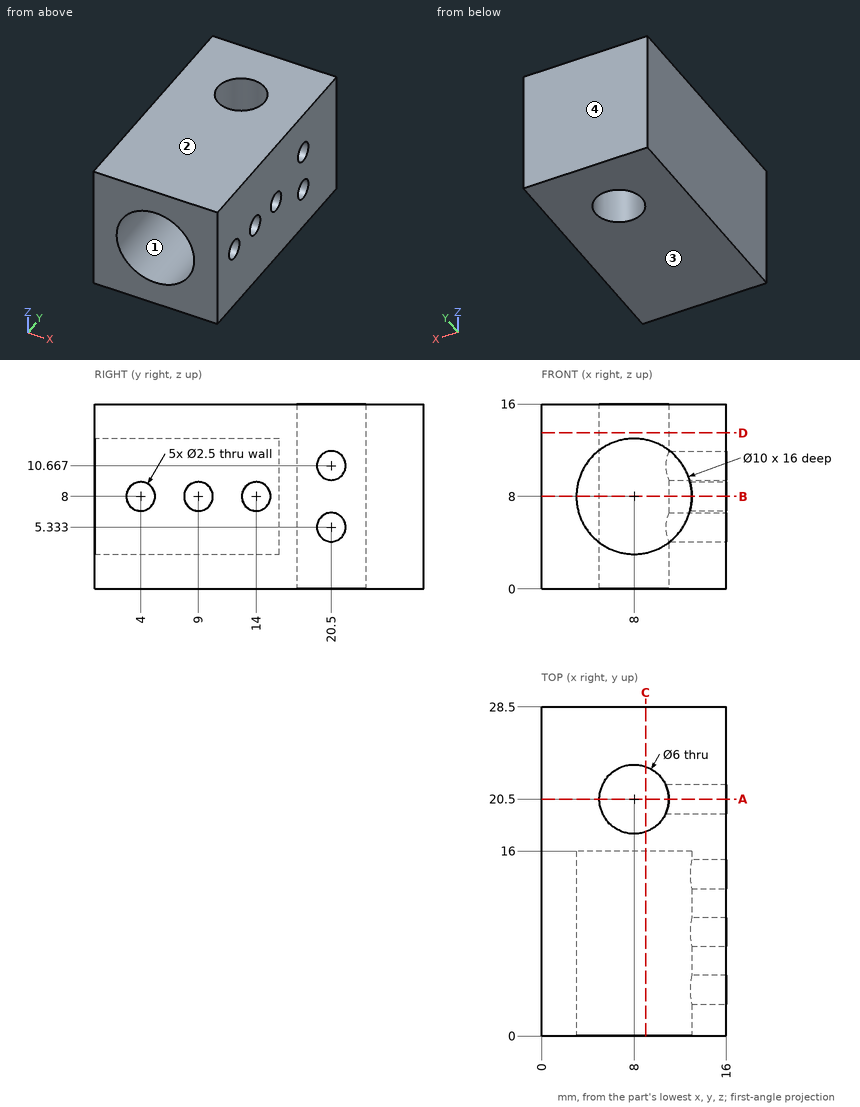
Study the drawing (mm; zero at the part's minimum x, y, z) and answer. Coordinates: 2 decimals unless noted, no trailing zeros. Write each loop counter-clockwise with the first axis right and the second up, starting at its lowest first coordinate (ties: lowest second). Pieces come first, ordered by that corner, then holes.
Q1. A cutting plane is placed at D-D, the plane z = 13.5. Give the vertices of the cut face in (x, y).
Q2. Each of these flat-tipped pins is pushed along its axis until it touches: pin 1 Ø1.5 at (y, z) = (9, 8) entering from +X; pin 2 Ø6 at (x, z) = (8, 8) entering from -Y; pin 3 Ø2 at (y, z) = (20.5, 10.67) entering from +X; pin 4 Ø3.5 at (x, y) = (8, 20.5) entering from -Z. Where does it stop, or does it pass through?
Q3. Determine the mould class of the marked faces 1, 2, 3 and 4 for opening direction Z: released by +Z, released by -Z, zero draft, split by the parting line, or undercut.
Q4. A cutting plane is placed at C-C, the plane x = 9. Give the vertices of the cut face in (y, z), then the cut area to 3 significant figures.
Q5. A cutting plane is placed at B-B, the plane z = 8. Give the vertices of the cut face in (x, y).
Q6. A cutting plane is placed at A-A, the plane y = 20.5. Give the vertices of the cut face in (x, z).
Q7. Find the intervals of material crossed by line 1 (Z direction, x = 13.7, y = 20.5); line 2 (Z direction, x = 7.75, y = 2); line 3 (Y direction, x = 5.75, z = 4.75) (1 decimal), in increasing order.
Findings below:
1. outline: (0, 0) - (16, 0) - (16, 28.5) - (0, 28.5) - close; hole circle Ø6 at (8, 20.5)
2. pin 1: stops at x = 3.06
2. pin 2: stops at y = 16
2. pin 3: stops at x = 5.17
2. pin 4: passes through
3. face 1: undercut
3. face 2: released by +Z
3. face 3: released by -Z
3. face 4: zero draft
4. outline: (0, 0) - (17.67, 0) - (17.67, 16) - (0, 16) - (0, 12.9) - (16, 12.9) - (16, 3.1) - (0, 3.1) - close; (23.33, 0) - (28.5, 0) - (28.5, 16) - (23.33, 16) - close
4. area: 209 mm2
5. outline: (0, 0) - (3, 0) - (3, 16) - (13, 16) - (13, 15.25) - (16, 15.25) - (16, 28.5) - (0, 28.5) - close; (13, 0) - (16, 0) - (16, 2.75) - (13, 2.75) - close; (13, 5.25) - (16, 5.25) - (16, 7.75) - (13, 7.75) - close; (13, 10.25) - (16, 10.25) - (16, 12.75) - (13, 12.75) - close; hole circle Ø6 at (8, 20.5)
6. outline: (0, 0) - (5, 0) - (5, 16) - (0, 16) - close; (11, 0) - (16, 0) - (16, 4.08) - (11, 4.08) - close; (11, 6.58) - (16, 6.58) - (16, 9.42) - (11, 9.42) - close; (11, 11.92) - (16, 11.92) - (16, 16) - (11, 16) - close
7. line 1: z = 0 to 4.08, 6.58 to 9.42, 11.92 to 16
7. line 2: z = 0 to 3.01, 12.99 to 16
7. line 3: y = 16 to 18.5, 22.5 to 28.5
